For this review, take the finished solid that the model builds, in its own axes (mm). A direction names the side the tool comes from. Round coordinates to 2 decimals unless told otherwise and drop trailing zeros. Loops run counter-clockwise (first coordinate to the right, second up) from the corner with the lowest first, then second, coordinate; pieces in that order, holes last. Notation, with made-up numbers: (-7.75, 41.25) -> (19.25, 41.25) arc R21 ccw to (19.25, 77.25) -> close; hole circle Ø5 at (66, 58). An arc over 180 degrees is marked (long way). One line per question, with ' | ' between items. Start each with the question number.
1. Draft analysis for pull direction Y (two halves, no side actions). For faces 3 (the face through (1.778, 23, 56)), 4 (the face through (55.46, 0, 5)), state which applies: pulls with the +Y half, pulls with the -Y half, needs draft (parallel to the pull), parting line crosses it, or undercut.
2. Consider section C-C (x = 8). Write out the cut boundary in (y, z).
3. For pin 1 Ø1.5 at (y, z) = (16.5, 12) entering from +X; pin 2 Ø2 at (x, z) = (45.5, -11) entering from +Y; pin 3 Ø5 at (x, y) = (35, -17.5) entering from -Z; pin 4 Ø3 at (x, y) = (53, 21.5) entering from +Z, all flat-tipped, find the tip position at first contact; note any pin that passes through.
4. For faces 1 (the face through (58, 0, -3.429)), 2 (the face through (59.88, 4, 0)), list the 3-axis set-ups (+Z, -Z, +X, -X, +Y, -Y) from which the entire face can be reached by the end or side of a thin tool; tool diameter is ignored.
5. Wall thickness on line 1 along Z through (x, y) = (17, 2); line 2 along Y through (x, z) = (51, 5); line 3 along Z through (x, y) = (14.5, -6.5): over which ranges is each line inside the solid? List them lowest first.
```python
from build123d import *

# Parameters (mm, degrees)
F3_R     = 21.082
F3_W     = 6.858
F3_H     = 6.858
F4_DEPTH = 16.3195
F5_DEPTH = 54.356


with BuildPart() as f1:
    # F0 (on Front) → F1 (revolve)
    with BuildSketch(Plane.XZ):
        with BuildLine():
            Line((60.325, 0), (63.5, 0))
            ThreePointArc((63.5, 0), (45.5255587555, 44.2681996472), (1.778, 63.4751031193))
            Line((1.778, 63.4751031193), (1.778, 60.2987922018))
            ThreePointArc((1.778, 60.2987922018), (33.9600417382, 49.8580102906), (55.4598304439, 23.7342122711))
            ThreePointArc((55.4598304439, 23.7342122711), (59.0961923331, 12.113862998), (60.325, 0))
        make_face()
        with BuildLine():
            Line((55.4598304439, 0), (60.325, 0))
            ThreePointArc((60.325, 0), (59.0961923331, 12.113862998), (55.4598304439, 23.7342122711))
            Line((55.4598304439, 23.7342122711), (55.4598304439, 0))
        make_face()
    revolve(axis=Axis((32.639, 0, 0), (1, 0, 0)))

    # F3 (on offset) → F4 (cut)
    with BuildSketch(Plane.YZ.offset(76.2)):
        Circle(F3_R)
        Rectangle(F3_W, F3_H, mode=Mode.SUBTRACT)
    extrude(amount=-F4_DEPTH, mode=Mode.SUBTRACT)

    # F3 (on offset) → F5 (cut)
    with BuildSketch(Plane.YZ.offset(76.2)):
        Rectangle(F3_W, F3_H)
    extrude(amount=-F5_DEPTH, mode=Mode.SUBTRACT)


solid = f1.part
```
Answer block:
1) face 3: needs draft | face 4: undercut
2) outline: circle Ø125.99 at (0, 0); hole circle Ø119.58 at (0, 0)
3) pin 1: stops at x = 59.9 | pin 2: stops at y = 43.97 | pin 3: stops at z = -51.87 | pin 4: stops at z = 30.5
4) face 1: +X, -X | face 2: +Z, -Z, +X, +Y, -Y
5) line 1: z = -61.15 to -57.85, 57.85 to 61.15 | line 2: y = -37.5 to -31.83, 31.83 to 37.5 | line 3: z = -61.48 to -58.19, 58.19 to 61.48
